Solid Edge part; units mm, degrees
sketch "Sketch1" plane through (0, 0, 0) normal (0, 0, 1) x (1, 0, 0)
  circle A0 centre (-68.9258, 50.0648) radius 125
extrude "Protrusion1" add sketch "Sketch1" along normal blind 10
sketch "Sketch2" plane through (-68.9258, 50.0648, 10) normal (0, 0, 1) x (1, 0, 0)
  circle A0 centre (0, 105) radius 5
extrude "Cutout1" cut sketch "Sketch2" against normal through all
pattern_circular "Pattern1" count 10 over 360 about axis through (-68.9258, 50.0648, 10) along (0, 0, -1) of "Cutout1"
sketch "Sketch3" plane through (-68.9258, 50.0648, 10) normal (0, 0, 1) x (1, 0, 0)
  circle A0 centre (0, 0) radius 25
extrude "Cutout2" cut sketch "Sketch3" against normal through all
Can you work these out from the model? Positions are in its coordinate system, mm. Coordinates: 2 decimals unless noted, no trailing zeros. Write each loop counter-clockwise with the first axis right and the second up, starting at its lowest first coordinate (ties: lowest second). Pieces come first, ordered by that corner, then holes. Notation, with made-up numbers: (-11.75, -27.75) - (11.25, -27.75) arc R29 ccw to (11.25, -4.75) - close; hole circle Ø4 at (2, 53). An arc over 180 degrees is marked (long way). Return JSON: item names as keys, results as strings.
Q1. If we section it at D-D (y = 125.5): Please give me the cut outline in (x, z), then the cut area to 3 significant figures.
Computed values:
{"outline": "(-168.6, 0) - (30.75, 0) - (30.75, 10) - (-168.6, 10) - close", "area": "1,990 mm2"}
Q2. If we section it at A-A (y = 43.5): Please give me the cut outline in (x, z), then the cut area to 3 significant figures.
Computed values:
{"outline": "(-193.75, 0) - (-93.05, 0) - (-93.05, 10) - (-193.75, 10) - close; (-44.8, 0) - (55.9, 0) - (55.9, 10) - (-44.8, 10) - close", "area": "2,010 mm2"}
Q3. Please list where these lines run through material, in increasing order: L1, parallel to X at y = -34.5, z = 1.25; L2, parallel to Y at x = -66.5, z = 9; L3, parallel to X at y = 64, z = 6. Write a range as from..to.
Computed values:
{"L1": "x = -160.98..-135.63, -125.66..-12.19, -2.22..23.13", "L2": "y = -74.91..-59.31, -50.56..25.18, 74.95..150.69, 159.44..175.04", "L3": "x = -193.15..-89.68, -48.17..55.3"}
Q4. Thinking about a two-plate mould opening in Y: for faces 1 (the flat face through (-43, 52, 10)), 2 (the cylindrical face through (-168.74, 87.51, 5.07)), 3 (the cylindrical face through (-193.805, 44.569, 4.93)), which applies, +Y half, -Y half, draft (parallel to the pull), parting line (faces both ways), or undercut?
Computed values:
{"face 1": "draft", "face 2": "undercut", "face 3": "parting line"}
Q5. I'm going to push flat-ended pins straight in: pin 1 Ø2 at (y, z) = (-49.5, 4) entering from +X; pin 2 Ø1.5 at (x, z) = (-162.5, 1.5) entering from +Y; pin 3 Ø2 at (x, z) = (-76.5, 5) entering from +Y. Where does each tip first touch, or does it pass through?
Computed values:
{"pin 1": "stops at x = 7.95", "pin 2": "stops at y = 133.78", "pin 3": "stops at y = 174.89"}
Q6. If we section it at C-C (x = -104.5): Please give me the cut outline in (y, z).
Computed values:
{"outline": "(-69.77, 0) - (169.9, 0) - (169.9, 10) - (-69.77, 10) - close"}
